Solid Edge part; units mm, degrees
sketch "Sketch1" plane through (0, 0, 0) normal (0, 0, 1) x (1, 0, 0)
  line L0 (-0.7217, 1.25) -> (0.7217, 1.25)
  line L1 (0.7217, 1.25) -> (1.4434, 0)
  line L2 (1.4434, 0) -> (0.7217, -1.25)
  line L3 (0.7217, -1.25) -> (-0.7217, -1.25)
  line L4 (-0.7217, -1.25) -> (-1.4434, 0)
  line L5 (-1.4434, 0) -> (-0.7217, 1.25)
  circle A0 centre (0, 0) radius 2.75
extrude "Protrusion1" add sketch "Sketch1" along normal blind 3
sketch "Sketch2" plane through (0, 0, 0) normal (0, -1, 0) x (1, 0, 0)
  line L0 (0, 0.8667) -> (1.4434, 1.7)
  line L1 (1.4434, 1.7) -> (2.75, 1.7)
  line L2 (2.75, 1.7) -> (2.75, 0)
  line L3 (2.75, 0) -> (1.5, 0)
  line L4 (1.5, 0) -> (1.5, -36.999)
  line L5 (1.5, -36.999) -> (1.5, -37) construction
  line L6 (1.5, -37) -> (1.5, -37) construction
  line L7 (1.5, -37) -> (1.5, -55)
  line L8 (0, -55) -> (1.5, -55)
revolve "RevolvedProtrusion_1" add sketch "Sketch2" angle 360 about axis through (0, 0, 2.3333) along (0, 0, -1)
cosmetic_thread "Thread_1" thread depth 17.999
sketch "Sketch3" plane through (0, 0, 0) normal (0, -1, 0) x (1, 0, 0)
  line L0 (0, 4) -> (1.435, 4)
  line L1 (1.435, 4) -> (1.435, 3)
  line L2 (1.435, 3) -> (0, 2.1715)
revolve "RevolvedCutout_1" cut sketch "Sketch3" angle 360 about axis through (0, 0, 7.1999) along (0, 0, 1)
fillet "Round_1" radius 0.3 1 edges at (-2.75, 0, 3)
sketch "Sketch4" plane through (0, 0, 0) normal (0, -1, 0) x (1, 0, 0)
  line L0 (1.5, 0) -> (1.8, 0)
  arc A0 (1.7101, -0.0562) -> (1.8, 0) centre (1.8, -0.1) cw
  line L1 (1.5101, -0.4662) -> (1.7101, -0.0562)
  arc A1 (1.5101, -0.4662) -> (1.5, -0.51) centre (1.6, -0.51) ccw
  line L2 (1.5, 0) -> (1.5, -0.51)
revolve "RevolvedProtrusion_2" add sketch "Sketch4" angle 360 about axis through (0, 0, -1.02) along (0, 0, 1)
chamfer "Chamfer_1" distance 0.2705 angle 45 1 edges at (-1.5, 0, -55)
properties material "Steel"
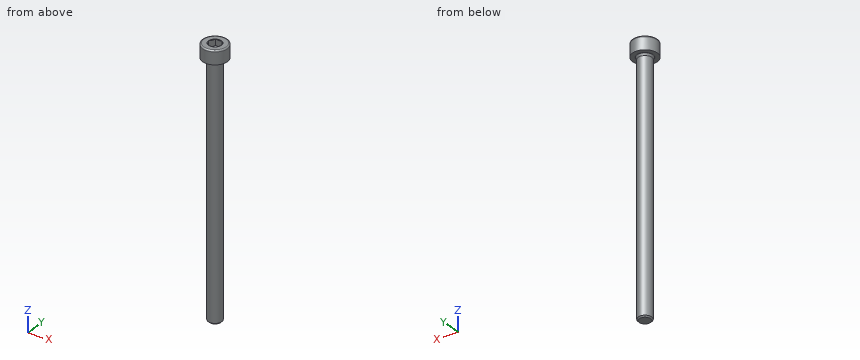
Part model, mm, in its own coordinate system. Coordinates: 2 decimals unless noted, no trailing zeros. Loops run counter-clockwise (first coordinate to the right, second up) from the corner with the lowest first, then second, coordinate; pieces in that order, holes last. Notation, with made-up numbers: (-24, 72) -> (-17, 72) arc R29 cw to (-17, 93) -> close; hole circle Ø9 at (26.25, 67). An arc over 180 degrees is marked (long way). Use a Markdown table: item, result. Add a question column.
Item 1: Flat gauge pins, fed straight in: P1, Ø0.7, axis at x = -0.5, z = 2.5, coming from the -Y side; P2, Ø2, axis at y = -0.5, z = -22.5, coming from the -X side. Where does each tip first touch, or does it go through?
Item 2: Probe probe 1 along Z at (x, y) = (-0.55, 1.7); probe 2 along X at (y, z) = (-0.05, -46.5); probe 3 along Z at (x, y) = (0.2, -1.7). List the from-to ranges inside material, lowest first.
Item 3: Band-saw the part on A-A on z = -15.5. Write the cut outline in (x, y).
Geometry says:
| question | item | result |
|---|---|---|
| 1 | P1 | y = -2.75 |
| 1 | P2 | x = -1.5 |
| 2 | probe 1 | 0 to 3 |
| 2 | probe 2 | -1.5 to 1.5 |
| 2 | probe 3 | -0.05 to 3 |
| 3 | outline | circle Ø3 at (0, 0) |
